Here's how the part is built. I have some questions about the finished solid (model axes, mm). Face numbers are marked on the shaded views. A direction names the side the tool comes from. Give positions to 0.01 mm unless a question says otherwise; leave off trailing zeros. Loops run counter-clockwise (first coordinate to the right, second up) from the corner with the lowest first, then second, coordinate; pieces in that order, holes last. Notation, with made-up numbers: M 39.25,79 L 65.25,79 A14 ccw 65.25,90 Z; hole C 88.25,29 d8. An arc over 180 degrees is marked long. Write item = value, one per line. Start each with the question number.
Autodesk Inventor part; units mm, degrees
ref_plane "Work Plane3" through (97.1697, -138.2024, -7.9168) normal (0, 0, 1) x (1, 0, 0)
ref_plane "Work Plane4" through (100.4, -134.9721, -1.51) normal (0, 0, -1) x (0, 1, 0)
ref_plane "Work Plane5" through (93.9197, -138.2024, -7.9168) normal (0, 0, 1) x (1, 0, 0)
ref_plane "Work Plane1" through (0, 0, 0) normal (0, 0, 1) x (1, 0, 0)
sketch "Sketch1" plane through (0, 0, 0) normal (0, 0, 1) x (1, 0, 0)
  line L0 (119.8428, -136.5657) -> (119.8428, -115.4866)
  arc A0 (119.8428, -115.4866) -> (104.8622, -116.0261) centre (112.3622, -116.0261) ccw
  line L1 (104.8622, -136.0261) -> (104.8622, -116.0261)
  arc A1 (104.8622, -136.0261) -> (119.8428, -136.5657) centre (112.3622, -136.0261) ccw
  circle A2 centre (117.3428, -116.0541) radius 0.5
  circle A3 centre (106.6428, -124.9791) radius 0.5
  circle A4 centre (106.6428, -127.5191) radius 0.5
  circle A5 centre (117.3428, -136.0541) radius 0.5
  arc A6 (103.3319, -124.86) -> (103.3319, -127.1923) centre (106.6319, -126.0261) ccw
  line L2 (103.3319, -124.86) -> (103.3319, -116.0261)
  arc A7 (121.3731, -115.4341) -> (103.3319, -116.0261) centre (112.3622, -116.0261) ccw
  line L3 (121.3731, -115.4341) -> (121.3731, -136.6182)
  arc A8 (103.3319, -136.0261) -> (121.3731, -136.6182) centre (112.3622, -136.0261) ccw
  line L4 (103.3319, -136.0261) -> (103.3319, -127.1923)
  arc A9 (121.8731, -115.4179) -> (102.8319, -116.0261) centre (112.3622, -116.0261) ccw
  line L5 (102.8319, -116.0261) -> (102.8319, -136.0261)
  arc A10 (102.8319, -136.0261) -> (121.8731, -136.6344) centre (112.3622, -136.0261) ccw
  line L6 (121.8731, -136.6344) -> (121.8731, -115.4179)
  point P0 (0, 0)
  point P1 (107.9, -107.4721)
  point P2 (107.9, -127.4721)
extrude "Extrusion1" add sketch "Sketch1" along normal blind 3 contours A1 L1 A0 L0 | A2 | A3 | A4 | A5
ref_plane "Work Plane3" through (97.1697, -138.2024, -7.9168) normal (0, 0, 1) x (1, 0, 0)
ref_plane "Work Plane4" through (100.4, -134.9721, -1.51) normal (0, 0, -1) x (0, 1, 0)
sketch "Sketch4" plane through (0, 0, 3) normal (0, 0, 1) x (1, 0, 0)
  line L0 (103.3319, -124.86) -> (103.3319, -116.0261)
  line L1 (103.3319, -136.0261) -> (103.3319, -127.1923)
  arc A0 (103.3319, -136.0261) -> (121.3731, -136.6182) centre (112.3622, -136.0261) ccw
  line L2 (121.3731, -115.4341) -> (121.3731, -136.6182)
  arc A1 (121.3731, -115.4341) -> (103.3319, -116.0261) centre (112.3622, -116.0261) ccw
  line L3 (103.3319, -124.86) -> (103.3319, -127.1923)
  circle A2 centre (112.3622, -136.0261) radius 6.35
  line L4 (119.8428, -136.5657) -> (119.8428, -115.4866)
  arc A3 (119.8428, -115.4866) -> (104.8622, -116.0261) centre (112.3622, -116.0261) ccw
  line L5 (104.8622, -116.0261) -> (104.8622, -136.0261)
  arc A4 (104.8622, -136.0261) -> (119.8428, -136.5657) centre (112.3622, -136.0261) ccw
  point P0 (0, 0)
extrude "Extrusion4" add sketch "Sketch4" against normal up to surface (4.51 mm away) contours L0 A1 L2 A0 L1 L3
sketch "Sketch5" plane through (121.3731, -136.6182, -1.51) normal (0, 0, -1) x (-1, 0, 0)
  line L0 (16.5109, 20.5921) -> (16.5109, 13.6117)
  line L1 (16.5109, 0.5921) -> (16.5109, 20.5921)
  arc A0 (1.5303, 0.0526) -> (16.5109, 0.5921) centre (9.0109, 0.5921) ccw
  line L2 (1.5303, 0.0526) -> (1.5303, 21.1316)
  arc A1 (16.5109, 20.5921) -> (1.5303, 21.1316) centre (9.0109, 20.5921) ccw
  line L3 (1.3303, 21.1388) -> (1.3303, 0.0454)
  arc A2 (1.3303, 0.0454) -> (16.7109, 0.5921) centre (9.0109, 0.5921) ccw
  line L4 (16.7109, 0.5921) -> (16.7109, 20.5921)
  arc A3 (16.7109, 20.5921) -> (1.3303, 21.1388) centre (9.0109, 20.5921) ccw
  point P0 (121.3731, 136.6182)
  dimension "d10" = 0.2
extrude "Extrusion5" cut sketch "Sketch5" against normal up to surface (1.51 mm away)
ref_plane "Work Plane5" through (93.9197, -138.2024, -7.9168) normal (0, 0, 1) x (1, 0, 0)
ref_plane "Work Plane6" through (93.9197, -138.2024, -7.9168) normal (0, 0, 1) x (1, 0, 0)
sketch "Sketch10" plane through (0, 0, 3) normal (0, 0, 1) x (1, 0, 0)
  line L0 (103.3319, -116.0261) -> (103.3319, -136.0261)
  arc A0 (103.3319, -124.86) -> (103.3319, -127.1923) centre (106.6319, -126.0261) ccw
  point P0 (0, 0)
  point P1 (103.3319, -135.2618)
extrude "Extrusion10" add sketch "Sketch10" against normal up to surface (4.51 mm away)
sketch "Sketch11" plane through (0, 0, 3) normal (0, 0, 1) x (1, 0, 0)
  circle A0 centre (124.0731, -115.3807) radius 1.5
  circle A1 centre (100.6319, -116.0261) radius 1.5
  circle A2 centre (124.0731, -136.6716) radius 1.5
  circle A3 centre (100.6319, -136.0261) radius 1.5
  line L0 (101.6319, -119.276) -> (100.632, -118.2761)
  line L1 (101.6319, -119.276) -> (101.6319, -132.7858)
  line L2 (101.6319, -132.7858) -> (100.6415, -133.7762)
  arc A4 (100.6415, -133.7762) -> (99.8748, -138.1449) centre (100.6319, -136.0261) ccw
  line L3 (99.8748, -138.1449) -> (102.4702, -140.1841)
  arc A5 (102.4702, -140.1841) -> (121.9777, -140.7888) centre (112.3622, -136.0261) ccw
  line L4 (124.6926, -138.8347) -> (121.9777, -140.7888)
  arc A6 (124.6926, -138.8347) -> (125.0601, -134.6496) centre (124.0731, -136.6716) ccw
  line L5 (125.0601, -134.6496) -> (123.0731, -132.4216)
  line L6 (123.0731, -132.4216) -> (123.0731, -119.6307)
  line L7 (125.0601, -117.4026) -> (123.0731, -119.6307)
  arc A7 (125.0601, -117.4026) -> (124.6926, -113.2176) centre (124.0731, -115.3807) ccw
  line L8 (124.6926, -113.2176) -> (121.9777, -111.2635)
  arc A8 (121.9777, -111.2635) -> (102.4702, -111.8682) centre (112.3622, -116.0261) ccw
  line L9 (99.8748, -113.9074) -> (102.4702, -111.8682)
  arc A9 (99.8748, -113.9074) -> (100.6319, -118.2761) centre (100.6319, -116.0261) ccw
  arc A10 (102.3319, -136.0261) -> (122.3731, -136.6502) centre (112.3622, -136.0261) ccw
  line L10 (102.3319, -136.0261) -> (102.3319, -116.0261)
  arc A11 (122.3731, -115.4021) -> (102.3319, -116.0261) centre (112.3622, -116.0261) ccw
  line L11 (122.3731, -115.4021) -> (122.3731, -136.6502)
  line L12 (102.3319, -136.0261) -> (102.3319, -116.0261)
  arc A12 (102.3319, -136.0261) -> (122.3731, -136.6502) centre (112.3622, -136.0261) ccw
  line L13 (122.3731, -115.4021) -> (122.3731, -136.6502)
  arc A13 (122.3731, -115.4021) -> (102.3319, -116.0261) centre (112.3622, -116.0261) ccw
  line L14 (102.8319, -116.0261) -> (102.8319, -136.0261)
  arc A14 (121.8731, -115.4179) -> (102.8319, -116.0261) centre (112.3622, -116.0261) ccw
  line L15 (121.8731, -136.6344) -> (121.8731, -115.4179)
  arc A15 (102.8319, -136.0261) -> (121.8731, -136.6344) centre (112.3622, -136.0261) ccw
  arc A16 (121.8731, -115.4179) -> (102.8319, -116.0261) centre (112.3622, -116.0261) ccw
  line L16 (102.8319, -116.0261) -> (102.8319, -136.0261)
  arc A17 (102.8319, -136.0261) -> (121.8731, -136.6344) centre (112.3622, -136.0261) ccw
  line L17 (121.8731, -136.6344) -> (121.8731, -115.4179)
  arc A18 (103.3319, -124.86) -> (103.3319, -127.1923) centre (106.6319, -126.0261) ccw
  line L18 (103.3319, -124.86) -> (103.3319, -116.0261)
  arc A19 (121.3731, -115.4341) -> (103.3319, -116.0261) centre (112.3622, -116.0261) ccw
  line L19 (121.3731, -115.4341) -> (121.3731, -136.6182)
  arc A20 (103.3319, -136.0261) -> (121.3731, -136.6182) centre (112.3622, -136.0261) ccw
  line L20 (103.3319, -136.0261) -> (103.3319, -127.1923)
  line L21 (101.6319, -119.276) -> (101.6319, -132.7858)
  line L22 (101.6319, -132.7858) -> (100.6415, -133.7762)
  circle A21 centre (100.6319, -136.0261) radius 2.25
  line L23 (99.8748, -138.1449) -> (102.4702, -140.1841)
  circle A22 centre (112.3622, -136.0261) radius 10.7303
  line L24 (121.9777, -140.7888) -> (124.6926, -138.8347)
  circle A23 centre (124.0731, -136.6716) radius 2.25
  line L25 (123.0731, -132.4216) -> (125.0601, -134.6496)
  line L26 (123.0731, -132.4216) -> (123.0731, -119.6307)
  line L27 (123.0731, -119.6307) -> (125.0601, -117.4026)
  line L28 (124.6926, -113.2176) -> (121.9777, -111.2635)
  circle A24 centre (112.3622, -116.0261) radius 10.7303
  line L29 (102.4702, -111.8682) -> (99.8748, -113.9074)
  circle A25 centre (100.6319, -116.0261) radius 2.25
  line L30 (100.6319, -118.2761) -> (101.6319, -119.276)
  circle A26 centre (124.0731, -115.3807) radius 2.25
  point P0 (0, 0)
ref_plane "Work Plane8" through (98.3819, -146.7565, -7.9168) normal (0, 0, 1) x (1, 0, 0)
extrude "Extrusion11" add sketch "Sketch11" against normal up to surface (10.9168 mm away) contours A0 A24 A26 A7 | A0 A24 A26 L11 A11 | A26 A11 A25 A24 A8 | A24 L8 A26 | A26 L7 L6 L5 A23 A22 L11 A24 | A24 L11 A26 | A26 A14 A25 A11 | A11 L11 A26 L15 A14 | A24 L15 A26 L11 | L11 A22 L15 A24 | A24 A25 L9 | A25 A14 L14 L10 A11 | A11 L10 A25 A24 A1 | A26 L15 A24 L19 A19 L18 L14 A25 A14 | A14 L15 A26 | A22 A23 L11 | L11 A23 L15 A22 | L15 A22 L19 A24 | A25 A24 A1 A9 | A25 L14 A14 | A23 A22 A2 A10 L11 | L11 A10 A23 A15 L15 | A23 A6 A22 A2 | L15 A23 A15 A21 L14 A22 L20 A20 L19 | A25 A24 L10 A22 A21 L2 L1 L0 | A25 L14 A24 L10 | L10 A24 A25 | L15 A15 A23 | A24 L14 A22 L10 | A23 A22 A5 A21 A10 | A10 A21 A15 A23 | A22 L14 A21 L10 | L10 A21 A22 | A24 L18 A18 L20 A22 L14 | A21 A22 A3 L10 A10 | A10 L10 A21 L14 A15 | A23 L4 A22 | A15 L14 A21 | A21 A22 A3 A4 | A22 L3 A21
sketch "Sketch13" plane through (101.6319, -132.7858, -7.9168) normal (0, 0, -1) x (-1, 0, 0)
  line L0 (-1.7, 5.5934) -> (-1.7, -3.2404)
  line L1 (-1.7, 5.5934) -> (-1.7, 7.9258)
  arc A0 (-19.7412, -3.8325) -> (-1.7, -3.2404) centre (-10.7303, -3.2404) ccw
  line L2 (-19.7412, 17.3517) -> (-19.7412, -3.8325)
  arc A1 (-1.7, 16.7596) -> (-19.7412, 17.3517) centre (-10.7303, 16.7596) ccw
  line L3 (-1.7, 7.9258) -> (-1.7, 16.7596)
  line L4 (-1.2, -3.2404) -> (-1.2, 5.5934)
  line L5 (-1.2, 5.5934) -> (-1.2, 7.9258)
  line L6 (-1.2, 7.9258) -> (-1.2, 16.7596)
  arc A2 (-1.2, 16.7596) -> (-20.2412, 17.3679) centre (-10.7303, 16.7596) ccw
  line L7 (-20.2412, 17.3679) -> (-20.2412, -3.8486)
  arc A3 (-20.2412, -3.8486) -> (-1.2, -3.2404) centre (-10.7303, -3.2404) ccw
  line L8 (-0.7, 5.5934) -> (-0.7, -3.2404)
  arc A4 (-20.7412, -3.8644) -> (-0.7, -3.2404) centre (-10.7303, -3.2404) ccw
  line L9 (-20.7412, -3.8644) -> (-20.7412, 17.3837)
  arc A5 (-0.7, 16.7596) -> (-20.7412, 17.3837) centre (-10.7303, 16.7596) ccw
  line L10 (-0.7, 16.7596) -> (-0.7, 7.9258)
  line L11 (-0.7, 7.9258) -> (-0.7, 5.5934)
  point P0 (101.6319, 132.7858)
  dimension "d31" = 0.5
  dimension "d32" = 0.5
extrude "Extrusion12" cut sketch "Sketch13" against normal blind 1 contours L8 A4 L9 A5 L10 L11
fillet "Fillet4" radius 1 4 edges at (112.0298, -105.301, 3) (101.6319, -126.0309, 3) (112.0298, -146.7513, 3) (123.0731, -126.0261, 3)
properties part number "battery_case_top"
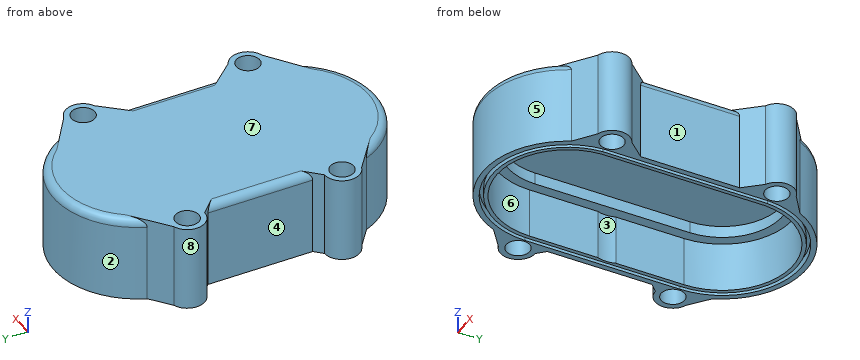
Q1. On a 3-axis mill with a long thin cutter (end or side, diameter ignored), from which of +Z, -Z, +X, -X, +Y, -Y can I reach the whole of each face in a straight line? I mean the marked faces 1, 2, 3, 4 and 5. Say none if no direction works.
Q2. Will these pins go through, and if not, where does the flat tip stop? pin 1 (5.5 mm diameter, centred on x = 113, y = -127, fed in from -Z); pin 2 (5 mm diameter, centred on y = -125, z = -5.5, fed in from -X); pin 3 (0.8 mm diameter, centred on y = -129.5, z = -7, fed in from +X).
Q3. If we section it at B-B, the plane z = -6.25: List the corners of the cut face in (x, y) for me, then the cut area to 3 significant figures.
Q4. If we section it at A-A, the plane z = 1.5: List the corners of the cut face in (x, y) for me.
Q5. If I drill on line 1 along X through (y, z) = (-132, -2.75); line 2 along Y through (x, z) = (101.25, -6.25); line 3 along Y through (x, z) = (123.25, -0.25), over which ranges is the centre line in solid material (lowest first)?
Q6. We'd pull the mould along X, two halves only. Please class the marked faces 6, 7 and 8: pulls with the +X half, pulls with the -X half, needs draft (parallel to the pull), parting line crosses it, or undercut.
Resolved:
q1.face_1 = +Z, -Z, +X
q1.face_2 = +Z, -Z, +Y
q1.face_3 = -Z
q1.face_4 = +Z, -Z, -X
q1.face_5 = +Z, -Z, -Y
q2.pin_1 = 0
q2.pin_2 = 101.63
q2.pin_3 = 123.07
q3.outline = M 99.87,-138.14 L 102.47,-140.18 A10.73 ccw 121.98,-140.79 L 124.69,-138.83 A2.25 ccw 125.06,-134.65 L 123.07,-132.42 L 123.07,-119.63 L 125.06,-117.4 A2.25 ccw 124.69,-113.22 L 121.98,-111.26 A10.73 ccw 102.47,-111.87 L 99.87,-113.91 A2.25 ccw 100.63,-118.28 L 101.63,-119.28 L 101.63,-132.79 L 100.64,-133.78 A2.25 ccw Z; hole C 100.63,-136.03 d3; hole C 100.63,-116.03 d3; hole M 103.33,-136.03 A9.03 ccw 121.37,-136.62 L 121.37,-115.43 A9.03 ccw 103.33,-116.03 L 103.33,-124.86 A3.5 ccw 103.33,-127.19 Z; hole C 124.07,-136.67 d3; hole C 124.07,-115.38 d3
q3.area = 207 mm²
q4.outline = M 99.87,-138.14 L 102.47,-140.18 A10.73 ccw 121.98,-140.79 L 124.69,-138.83 A2.25 ccw 125.06,-134.65 L 123.07,-132.42 L 123.07,-119.63 L 125.06,-117.4 A2.25 ccw 124.69,-113.22 L 121.98,-111.26 A10.73 ccw 102.47,-111.87 L 99.87,-113.91 A2.25 ccw 100.63,-118.28 L 101.63,-119.28 L 101.63,-132.79 L 100.64,-133.78 A2.25 ccw Z; hole C 100.63,-136.03 d3; hole C 100.63,-116.03 d3; hole C 124.07,-136.67 d3; hole C 124.07,-115.38 d3
q5.line_1 = 101.63 to 103.33, 121.37 to 123.07
q5.line_2 = -139.23 to -137.39, -134.66 to -133.17, -118.89 to -117.39, -114.66 to -112.83
q5.line_3 = -139.87 to -137.93, -135.42 to -132.62, -119.43 to -116.63, -114.13 to -112.18
q6.face_6 = undercut
q6.face_7 = needs draft
q6.face_8 = pulls with the -X half
